Geometry check sheet. Reference: drawing and pictorial views, mm from the part's lowest x, y, z. Round coordinates to 2 decimals unless told otherwise and drop trailing zeros. Loops run counter-clockwise (first coordinate to the right, second up) from the corner with the lowest first, then second, coordinate; pieces in that order, holes last. Notation, with made-up numbers: M -31,-16 L 2,-16 A10 cw 2,3 Z; hole C 89,-21 d10. An arc over 180 degrees is marked long. One line per question, with ' | ' between items. Start each with the question number.
(1) Section check A-A (y = 25). Record the boundary of the cut face in (x, z).
(2) Go/stop test with flat-tipped pins: P1, Ø12, axis at x = 18.5, y = 25.5, coming from the -Z side; P2, Ø12, axis at x = 23, z = 31.5, coming from the +Y side; P3, Ø1.5, axis at x = 27.5, z = 78, coming from the -Y side; P4, Ø5, axis at x = 21, y = 34, coming from the +Z side. Record where each tip stops, or that it passes through.
(3) Draft check along X on the marked faces 1 and 2. Enter one of: +X half, -X half, draft (parallel to the pull), parting line (faces both ways), or undercut.
(4) Section check C-C (z = 71). Record the boundary of the cut face in (x, y), and give its area (3 significant figures).
(5) Thickness scan on probe 1 along Y at (x, z) = (25, 90.5); probe 2 along X at (y, z) = (30, 65). Record the ranges inside material, lowest first. Write a range as [from, to].
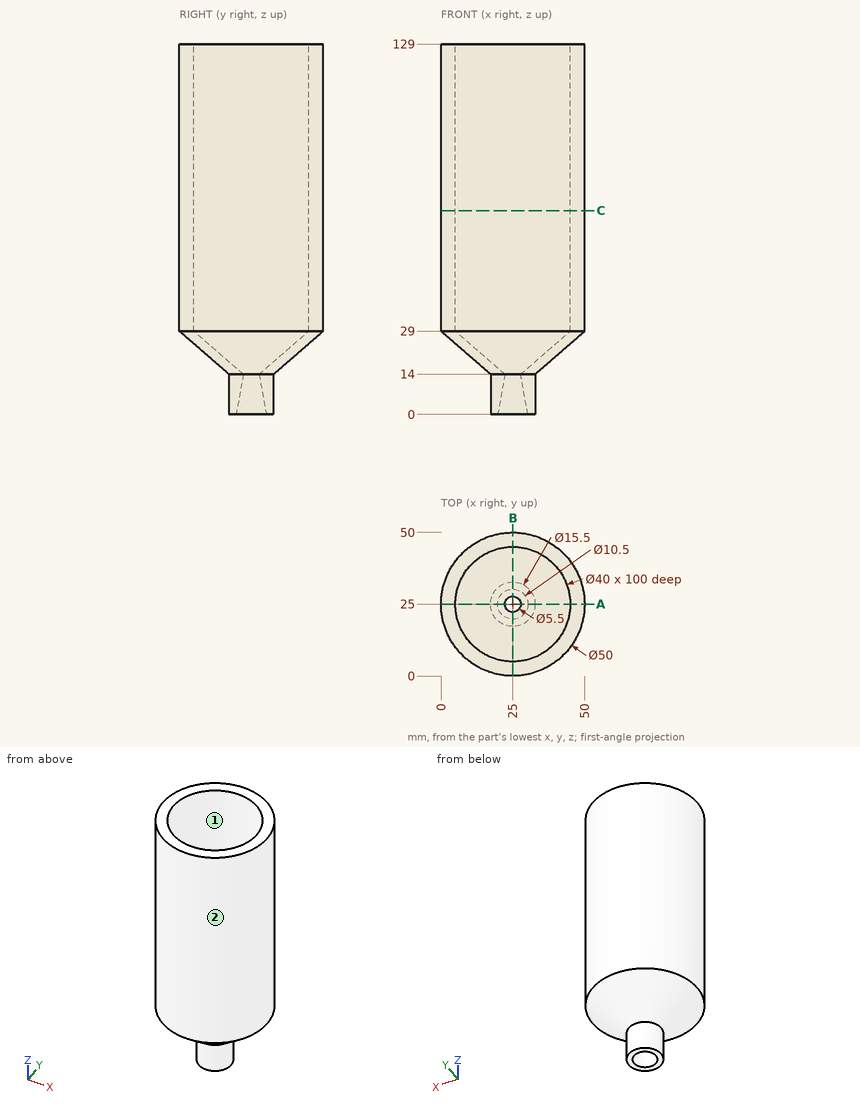
The answers:
1) outline: M 0,29 L 17.25,14 L 17.25,0 L 19.75,0 L 22.25,14 L 5,29 L 5,129 L 0,129 Z; M 27.75,14 L 30.25,0 L 32.75,0 L 32.75,14 L 50,29 L 50,129 L 45,129 L 45,29 Z
2) P1: z = 0 | P2: y = 50 | P3: y = 0.06 | P4: z = 22.35
3) face 1: undercut | face 2: parting line
4) outline: C 25,25 d50; hole C 25,25 d40 | area: 707 mm²
5) probe 1: [0, 5], [45, 50] | probe 2: [0.51, 5.64], [44.36, 49.49]
